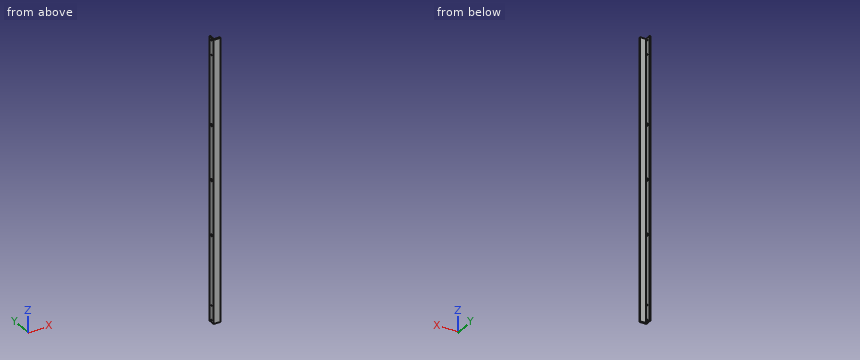
from build123d import *

# Parameters (mm, degrees)
BOSS_EXTRUDE1_DEPTH                  = 762
F_35_0_11_DIAMETER_HOLE1_D           = 2.794
F_17_64_0_26563_DIAMETER_HOLE1_D     = 6.747002
F_17_64_0_26563_DIAMETER_HOLE1_DEPTH = 10
F_17_64_0_26563_DIAMETER_HOLE1_TIP   = 2.027003899


with BuildPart() as part:
    # Sketch1 → Boss-Extrude1 (new body)
    with BuildSketch(Plane.XY):
        Polygon((0, 0), (19.05, 0), (19.05, 3.175), (3.175, 3.175), (3.175, 19.05), (0, 19.05), align=None)
    extrude(amount=BOSS_EXTRUDE1_DEPTH)

    # #35 (0.11) Diameter Hole1 (through all)
    with Locations(Plane(origin=(0, 9.525, 5.588), x_dir=(0, -1, 0), z_dir=(-1, 0, 0))):
        with Locations((0, 0), (0, 39.624), (0, 711.199), (0, 750.824)):
            Hole(F_35_0_11_DIAMETER_HOLE1_D / 2)

    # 17/64 (0.26563) Diameter Hole1
    with Locations(Plane(origin=(0, 9.525, 233.3625), x_dir=(0, -1, 0), z_dir=(-1, 0, 0))):
        with Locations((0, 0), (0, 147.6375), (0, 295.275)):
            Hole(F_17_64_0_26563_DIAMETER_HOLE1_D / 2, depth=F_17_64_0_26563_DIAMETER_HOLE1_DEPTH)
            with Locations((0, 0, -(F_17_64_0_26563_DIAMETER_HOLE1_DEPTH + F_17_64_0_26563_DIAMETER_HOLE1_TIP / 2))):  # 118° drill point
                Cone(0, F_17_64_0_26563_DIAMETER_HOLE1_D / 2, F_17_64_0_26563_DIAMETER_HOLE1_TIP, mode=Mode.SUBTRACT)


solid = part.part
Can you work these out from the model? Positions are in its coordinate system, mm. Coordinates: 2 decimals unless noted, no trailing zeros. Loops run counter-clockwise (first coordinate to the right, second up) from the corner with the lowest first, then second, coordinate; pieces in that order, holes last. Notation, with made-up numbers: (21.25, -5) - (69.25, -5) arc R29 cw to (69.25, 33) - close; hole circle Ø11 at (49, 57). An arc over 180 degrees is marked (long way). Answer as a JSON object with one key per item and string values. Group by question number.
Item 1: If we section it at B-B (x = 8): List the corners of the cut face in (y, z) for me (3 decimals), plus the area to 3 significant figures.
Item 2: If we section it at A-A (z = 415): List the corners of the cut face in (x, y) for me (3 decimals).
Item 3: For pin 1 (8 mm diameter, centred on y = 9.5, z = 354.5, fed in from +X) (3 decimals); pin 2 (1 mm diameter, centred on x = 11.5, z = 614.5, fed in from +Y) (3 decimals), each with a flat end and sliding along its axis, tell me the tip position at first contact or that it passes through.
Item 4: If I drill on L1, parallel to X at y = 10.25, z = 129 (3 decimals), over which ranges is the centre line in solid material (lowest first)? Write a range as from..to.
Returned:
{
 "1": {"outline": "(0, 0) - (3.175, 0) - (3.175, 762) - (0, 762) - close", "area": "2,420 mm²"},
 "2": {"outline": "(0, 0) - (19.05, 0) - (19.05, 3.175) - (3.175, 3.175) - (3.175, 19.05) - (0, 19.05) - close"},
 "3": {"pin 1": "stops at x = 3.175", "pin 2": "stops at y = 3.175"},
 "4": {"L1": "x = 0..3.175"}
}
